Part model, mm, in its own coordinate system. A direction names the side the tool comes from. Round coordinates to 2 decimals unless told otherwise and drop trailing zeros. Loops run counter-clockwise (first coordinate to the right, second up) from the corner with the lowest first, then second, coordinate; pieces in that order, holes last. Notation, with made-up numbers: (0, 30.25) -> (46, 30.25) arc R19 cw to (46, 34.25) -> close; hole circle Ø4 at (-8, 10.25). An arc over 180 degrees is marked (long way). Answer as CSV lines item,"result".
from build123d import *

# Parameters (mm, degrees)
BOSS_EXTRUDE1_DEPTH      = 10
SWEEP1_PROFILE_R         = 3.5
FILLET1_R                = 2
CHAMFER1_SIZE            = 1
FILLET1_OF_MIRROR1_R     = 2
CHAMFER1_OF_MIRROR1_SIZE = 1


with BuildPart() as part:
    # Sketch1 → Boss-Extrude1 (new body)
    with BuildSketch(Plane.XY):
        with BuildLine():
            Line((-13, 62.5), (-11, 61.25))
            Line((-11, 61.25), (-11, 62.5))
            Line((-11, 62.5), (-9, 61.25))
            Line((-9, 61.25), (-9, 62.5))
            Line((-9, 62.5), (-4, 62.5))
            Line((-4, 62.5), (-4, 4))
            Line((-4, 4), (-11.5, 4))
            Line((-11.5, 4), (-13, 2.5))
            Line((-13, 2.5), (-13, 2))
            ThreePointArc((-13, 2), (-12.414213562, 0.585786438), (-11, 0))
            Line((-11, 0), (-2, 0))
            ThreePointArc((-2, 0), (-0.585786438, 0.585786438), (0, 2))
            Line((0, 2), (0, 64.5))
            ThreePointArc((0, 64.5), (-0.585786438, 65.914213562), (-2, 66.5))
            Line((-2, 66.5), (-4, 66.5))
            Line((-4, 66.5), (-11, 66.5))
            ThreePointArc((-11, 66.5), (-12.414213562, 65.914213562), (-13, 64.5))
            Line((-13, 64.5), (-13, 62.5))
        make_face()
    extrude(amount=BOSS_EXTRUDE1_DEPTH)

    # Sweep1: sweep along a curve in space
    with BuildLine() as sweep1_path:
        Line((0, 9, 5), (8, 9, 5))
        ThreePointArc((8, 9, 5), (11.535533906, 10.464466094, 5), (13, 14, 5))
        Line((13, 14, 5), (13, 18, 5))
    # Sweep1 profile (on start of the path) → Sweep1 (sweep)
    with BuildSketch(Plane(origin=(0, 9, 5), x_dir=(0, 0, 1), z_dir=(1, 0, 0))):
        Circle(SWEEP1_PROFILE_R)
    sweep1 = sweep(path=sweep1_path.line)

    # Fillet1
    fillet1_edges = [part.edges().sort_by_distance(p)[0] for p in [
        (0, 9, 1.5),
    ]]
    fillet(fillet1_edges, radius=FILLET1_R)

    # Chamfer1
    chamfer1_edges = [part.edges().sort_by_distance(p)[0] for p in [
        (13, 18, 1.5),
    ]]
    chamfer(chamfer1_edges, length=CHAMFER1_SIZE)

    # Mirror1: Sweep1 across plane
    add(sweep1.mirror(Plane(origin=(0, 33.25, 0), x_dir=(0, 0, 1), z_dir=(0, -1, 0))))

    # Fillet1 of Mirror1
    fillet1_of_mirror1_edges = [part.edges().sort_by_distance(p)[0] for p in [
        (0, 57.5, 1.5),
    ]]
    fillet(fillet1_of_mirror1_edges, radius=FILLET1_OF_MIRROR1_R)

    # Chamfer1 of Mirror1
    chamfer1_of_mirror1_edges = [part.edges().sort_by_distance(p)[0] for p in [
        (13, 48.5, 1.5),
    ]]
    chamfer(chamfer1_of_mirror1_edges, length=CHAMFER1_OF_MIRROR1_SIZE)


solid = part.part
Q1. Saw through at B-B, the plane y = 51. Write the cut outline in (x, z).
Geometry results:
outline,"(-4, 0) -> (0, 0) -> (0, 10) -> (-4, 10) -> close; circle Ø7 at (13, 5)"
Q2. Drop flat-ended pins along their axis: P1, Ø1.5, axis at y = 19, z = 3.5, coming from the -X side; P2, Ø4, axis at x = 5, z = 1.5, coming from the -Y side; P3, Ø5, axis at y = 4, z = 5, coming from the +X side. Give the stop position or say it passes through.
Geometry results:
P1,"x = -4"
P2,"y = 5.84"
P3,"x = 12"
Q3. Which spindle directions (+Z, -Z, +X, -X, +Y, -Y) get a long thin tool onto all of the face, cutting with end or side? Do faces 4 (the face through (-12.2, 3.3, 4.9)), 5 (the face through (13, 49, 2)), 6 (the face through (-7, 62.5, 5)), 7 (the face through (0, 63.2, 4.9)). Say none if no direction does.
Geometry results:
face 4,"+Z, -Z, -X"
face 5,"none"
face 6,"+Z, -Z"
face 7,"+X, +Y"
Q4. Drill centre lines: line 1 along Y through (x, z) = (-8.5, 6); line 2 along X through (y, z) = (28.5, 3.5); line 3 along X through (y, z) = (53.5, 3.75). Where is each one in solid material? Low to high.
Geometry results:
line 1,"0 to 4, 62.5 to 66.5"
line 2,"-4 to 0"
line 3,"-4 to 0.49, 9.41 to 16.21"
Q5. Saw through at A-A, the plane x = -8.25. Write the cut outline in (y, z), then the cut area to 3 significant figures.
Geometry results:
outline,"(0, 0) -> (4, 0) -> (4, 10) -> (0, 10) -> close; (62.5, 0) -> (66.5, 0) -> (66.5, 10) -> (62.5, 10) -> close"
area,"80.0 mm2"
Q6. Saw through at C-C, the plane y = 36.5. Write the cut outline in (x, z).
Geometry results:
outline,"(-4, 0) -> (0, 0) -> (0, 10) -> (-4, 10) -> close"
Q7. Two-plate mould, pull along X, no slides. Class faces 1 (the face through (-0.6, 0.57, 4.93)), 2 (the face through (13, 48.5, 5)), 3 (the face through (-10.01, 61.88, 4.93)): pulls with the +X half, pulls with the -X half, needs draft (parallel to the pull), parting line crosses it, or undercut.
Geometry results:
face 1,"pulls with the +X half"
face 2,"needs draft"
face 3,"undercut"
